Here's the drawing with two shaded views (mm, measured from the low corner). I have some questions. A direction names the side the tool comes from. Give positions to 0.01 mm unless a question says otherwise; leave off trailing zeros. Write each loop counter-clockwise with the first axis right and the second up, starting at its lowest first coordinate (ties: lowest second). Pieces come first, ordered by that corner, then holes. Notation, with made-up numbers: (-14, -5) -> (23, -5) arc R24 cw to (23, 6) -> close; hole circle Ø10 at (-3.75, 0). An arc over 180 degrees is marked (long way). Put each result on its own line as item: value. Start each with the question number.
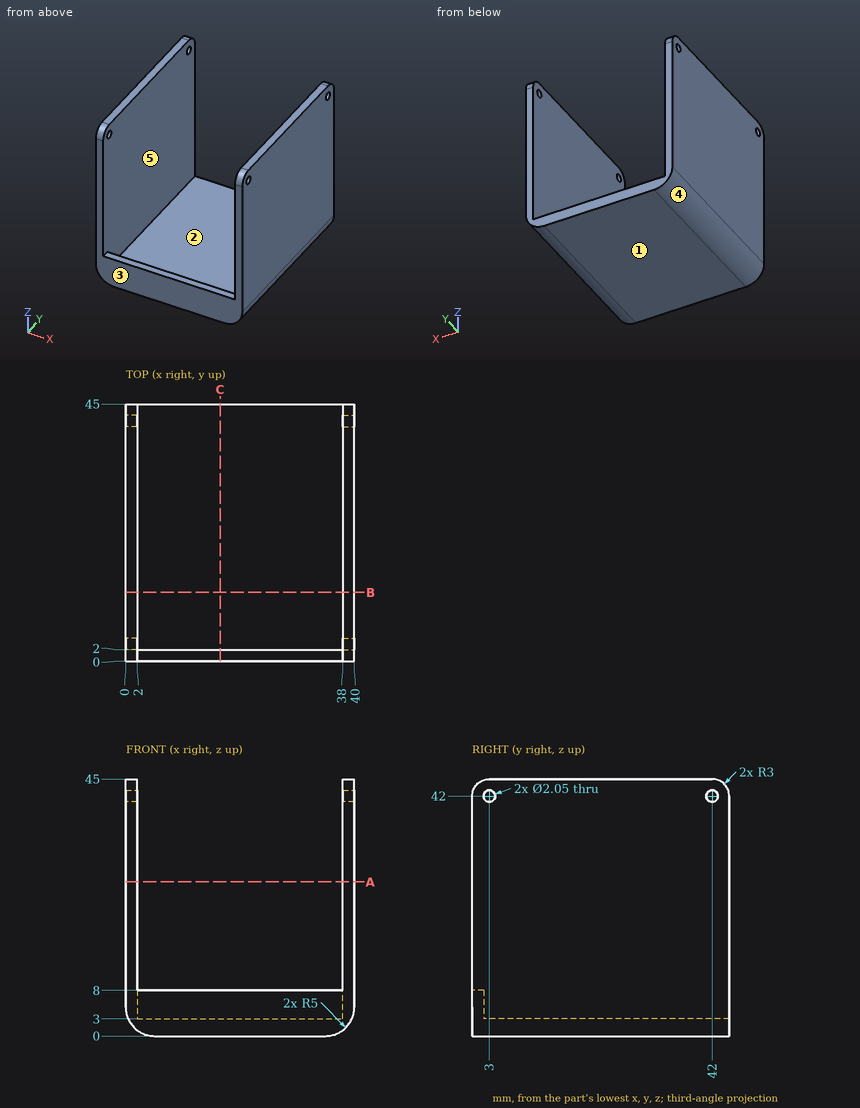
1) I need wall thicknesses on probe 1 along Y at (x, z) = (38.85, 42) (3 decimals); probe 2 along X at (y, z) = (8, 15.5); probe 3 along Z at (x, y) = (17.5, 4). Which ranges of each line are inside material? Lowest first, please.
2) I'm going to push flat-ended pins straight in: pin 1 Ø2.5 at (x, z) = (24, 6.5) entering from +Y; pin 2 Ø1 at (x, y) = (19, 0.5) entering from +Z; pin 3 Ø5 at (x, y) = (11.5, 31.5) entering from +Z. Where does each tip first touch, or does it pass through?
3) I want a section at A-A, the plane z = 27. Write out the boundary of the cut face in (x, y).
4) Which directions (+Z, -Z, +X, -X, +Y, -Y) give clear straight access to the entire face, cutting with the end or side of a thin tool? Please do the marked faces 1 and 2.
5) Thinking about a two-plate mould opening in X: for the marked faces 3, 4 and 5, which applies, released by +X, released by -X, zero draft, split by the parting line, or undercut?
6) I want a section at B-B, the plane y = 12. Write out the boundary of the cut face in (x, z).
7) I want a section at C-C, the plane x = 16.5. Write out the boundary of the cut face in (y, z), and give its area (3 significant figures).
Established:
1. probe 1: y = 0 to 1.975, 4.025 to 40.975, 43.025 to 45
1. probe 2: x = 0 to 2, 38 to 40
1. probe 3: z = 0 to 3
2. pin 1: stops at y = 2
2. pin 2: stops at z = 8
2. pin 3: stops at z = 3
3. outline: (0, 0) -> (2, 0) -> (2, 45) -> (0, 45) -> close; (38, 0) -> (40, 0) -> (40, 45) -> (38, 45) -> close
4. face 1: -Z, +X, -X, +Y, -Y
4. face 2: +Z, +Y
5. face 3: zero draft
5. face 4: released by -X
5. face 5: undercut
6. outline: (0, 5) arc R5 ccw to (5, 0) -> (35, 0) arc R5 ccw to (40, 5) -> (40, 45) -> (38, 45) -> (38, 3) -> (2, 3) -> (2, 45) -> (0, 45) -> close
7. outline: (0, 0) -> (45, 0) -> (45, 3) -> (2, 3) -> (2, 8) -> (0, 8) -> close
7. area: 145 mm2
